Geometry: see drawing. Coordinates: mm, zero at the bounding-box minimum. A direction names the side the tool comes from. Give positions to 0.01 mm unless a question says otherwise; leave off trailing zeros. Order: outer loops, then holes, each group sorted by start corner. A loop starts at its lowest first (then second) coordinate and runs counter-clockwise, first axis right, second up. Notation, with made-up numbers: M -29,-23.5 L 11,-23.5 A22 ccw 11,9.5 Z; hole C -27.5,-37 d8. An arc over 180 degrees is marked long. Use a Markdown table: item, result.
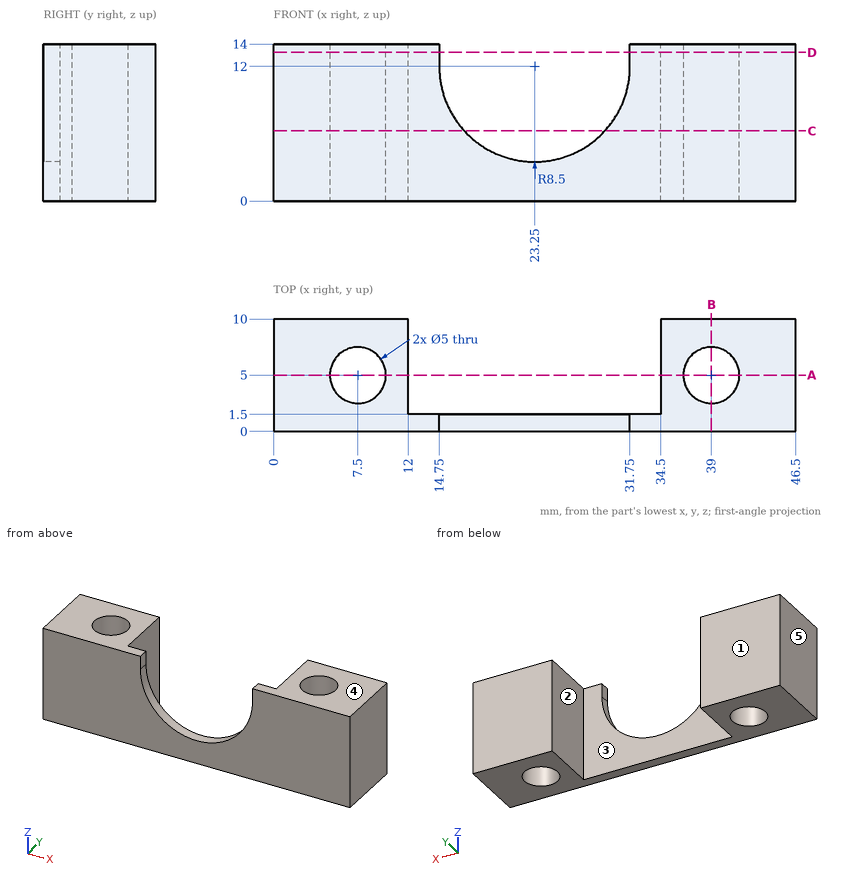
1) Cut plane C-C on z = 6.25. Return loops of the section in (x, y), and give its area (3 significant figures).
Response values:
| item | result |
|---|---|
| outline | M 0,0 L 16.99,0 L 16.99,1.5 L 12,1.5 L 12,10 L 0,10 Z; M 29.51,0 L 46.5,0 L 46.5,10 L 34.5,10 L 34.5,1.5 L 29.51,1.5 Z; hole C 7.5,5 d5; hole C 39,5 d5 |
| area | 216 mm² |
2) Reachability of the marked faces 1 and 2 from +Z, -Z, +X, -X, +Y, -Y: full face, straight path, thin tool, end or side. Return the list, or none.
Response values:
| item | result |
|---|---|
| face 1 | +Z, -Z, +X, -X, +Y |
| face 2 | +Z, -Z, +Y |
3) Cut plane B-B on x = 39. Return loops of the section in (y, z).
Response values:
| item | result |
|---|---|
| outline | M 0,0 L 2.5,0 L 2.5,14 L 0,14 Z; M 7.5,0 L 10,0 L 10,14 L 7.5,14 Z |
4) Material intervals for line 1 (X direction, y = 8.5, z = 10); line 2 (Y direction, x = 7.5, z = 5.75); line 3 (X direction, y = 5.25, z = 4.75), sorted ascending. Write a range as from..to.
Response values:
| item | result |
|---|---|
| line 1 | x = 0..12, 34.5..46.5 |
| line 2 | y = 0..2.5, 7.5..10 |
| line 3 | x = 0..5.01, 9.99..12, 34.5..36.51, 41.49..46.5 |
5) First-contact query: pin 1 Ø3 at (x, y) = (7.5, 5) entering from -Z; pin 2 Ø7 at (x, z) = (20, 6) entering from +Y. Flat tips, straight axial feed; report the tip coordinate or a pass-through.
Response values:
| item | result |
|---|---|
| pin 1 | passes through |
| pin 2 | stops at y = 1.5 |
6) Cut plane A-A on y = 5. Return loops of the section in (x, z).
Response values:
| item | result |
|---|---|
| outline | M 0,0 L 5,0 L 5,14 L 0,14 Z; M 10,0 L 12,0 L 12,14 L 10,14 Z; M 34.5,0 L 36.5,0 L 36.5,14 L 34.5,14 Z; M 41.5,0 L 46.5,0 L 46.5,14 L 41.5,14 Z |
7) Cut plane D-D on z = 13.25. Return loops of the section in (x, y), and give its area (3 significant figures).
Response values:
| item | result |
|---|---|
| outline | M 0,0 L 14.75,0 L 14.75,1.5 L 12,1.5 L 12,10 L 0,10 Z; M 31.75,0 L 46.5,0 L 46.5,10 L 34.5,10 L 34.5,1.5 L 31.75,1.5 Z; hole C 7.5,5 d5; hole C 39,5 d5 |
| area | 209 mm² |
8) Mould query, pull axis X, two halves, no side actions, for the marked faces 3, 4 and 5. Classes: released by +X, released by -X, zero draft, split by the parting line, or undercut.
Response values:
| item | result |
|---|---|
| face 3 | undercut |
| face 4 | zero draft |
| face 5 | released by -X |
